from build123d import *

# Parameters (mm, degrees)
F0_W     = 60
F0_H     = 8
F1_DEPTH = 5
F2_R     = 2.3
F2_R_2   = 2.25
F3_DEPTH = 5.001
F4_SIZE  = 1


with BuildPart() as f1:
    # F0 (on Top) → F1 (new body)
    with BuildSketch(Plane.XY):
        with Locations((0.770761, -3.362608)):
            Rectangle(F0_W, F0_H)
    extrude(amount=F1_DEPTH)

    # F2 (on face) → F3 (cut, through all)
    with BuildSketch(Plane.XY.offset(5)):
        with Locations((-8.229239, -3.362608)):
            Circle(F2_R)
        with Locations((9.770761, -3.362608)):
            Circle(F2_R_2)
        with Locations((25.770761, -3.362608)):
            Circle(F2_R_2)
        with Locations((-24.229239, -3.362608)):
            Circle(F2_R_2)
    extrude(amount=-F3_DEPTH, mode=Mode.SUBTRACT)

    # F4
    f4_edges = [f1.edges().sort_by_distance(p)[0] for p in [
        (0.770761, 0.637392, 5),
    ]]
    chamfer(f4_edges, length=F4_SIZE)


solid = f1.part
Geometry check sheet. Reference: the model listing, model coordinates, mm. Give positions to 0.01 mm unless a question says otherwise; leave off trailing zeros. Write each loop counter-clockwise with the first axis right and the second up, starting at its lowest first coordinate (ties: lowest second). Pieces come first, ordered by that corner, then holes. Notation, with made-up numbers: (85, 76.5) - (103, 76.5) arc R32 ccw to (103, 108.5) - close; hole circle Ø1 at (-7, 87). An arc over 180 degrees is marked (long way). Put each result on its own line as item: value.
1. Sectioned sample at B-B, the plane y = -2.5. Enter the section's corners in (x, z), plus the area to 3 significant figures.
Ans:
outline: (-29.23, 0) - (-26.31, 0) - (-26.31, 5) - (-29.23, 5) - close; (-22.15, 0) - (-10.36, 0) - (-10.36, 5) - (-22.15, 5) - close; (-6.1, 0) - (7.69, 0) - (7.69, 5) - (-6.1, 5) - close; (11.85, 0) - (23.69, 0) - (23.69, 5) - (11.85, 5) - close; (27.85, 0) - (30.77, 0) - (30.77, 5) - (27.85, 5) - close
area: 216 mm²
2. Thickness scan on line 1 (X direction, y = -3.5, z = 2.7); line 2 (Y direction, x = 26, z = 0.3); line 3 (X direction, y = -2.5, z = 2.7). Record the ranges inside material, lowest first.
Ans:
line 1: x = -29.23 to -26.48, -21.98 to -10.53, -5.93 to 7.52, 12.02 to 23.52, 28.02 to 30.77
line 2: y = -7.36 to -5.6, -1.12 to 0.64
line 3: x = -29.23 to -26.31, -22.15 to -10.36, -6.1 to 7.69, 11.85 to 23.69, 27.85 to 30.77
3. Sectioned sample at A-A, the plane x = -10. Enter the section's corners in (y, z).
Ans:
outline: (-7.36, 0) - (-4.83, 0) - (-4.83, 5) - (-7.36, 5) - close; (-1.89, 0) - (0.64, 0) - (0.64, 4) - (-0.36, 5) - (-1.89, 5) - close
4. Sectioned sample at C-C, the plane z = 0.8. Enter the section's corners in (x, y), plus the area to 3 significant figures.
Ans:
outline: (-29.23, -7.36) - (30.77, -7.36) - (30.77, 0.64) - (-29.23, 0.64) - close; hole circle Ø4.5 at (-24.23, -3.36); hole circle Ø4.6 at (-8.23, -3.36); hole circle Ø4.5 at (9.77, -3.36); hole circle Ø4.5 at (25.77, -3.36)
area: 416 mm²
5. Draft check along X on faces 1 (the flat face through (30.771, -3, 2)), 2 (the cylindrical face through (7.523, -3.264, 2.535)), 3 (the cylindrical face through (-10.527, -3.261, 2.535)), 4 (the flat face through (0, 0.637, 2)). Enter one of: +X half, -X half, draft (parallel to the pull), parting line (faces both ways), or undercut.
Ans:
face 1: +X half
face 2: undercut
face 3: undercut
face 4: draft
6. Sectioned sample at D-D, the plane x = -24.5. Enter the section's corners in (y, z), plus the area to 3 significant figures.
Ans:
outline: (-7.36, 0) - (-5.6, 0) - (-5.6, 5) - (-7.36, 5) - close; (-1.13, 0) - (0.64, 0) - (0.64, 4) - (-0.36, 5) - (-1.13, 5) - close
area: 17.2 mm²
7. Go/stop test with a flat-tipped pin: pin 1 (3.5 mm diameter, centred on x = 9.77, y = -3.36, fed in from -Z). Record where the tip stops, or that it passes through.
Ans:
pin 1: passes through
